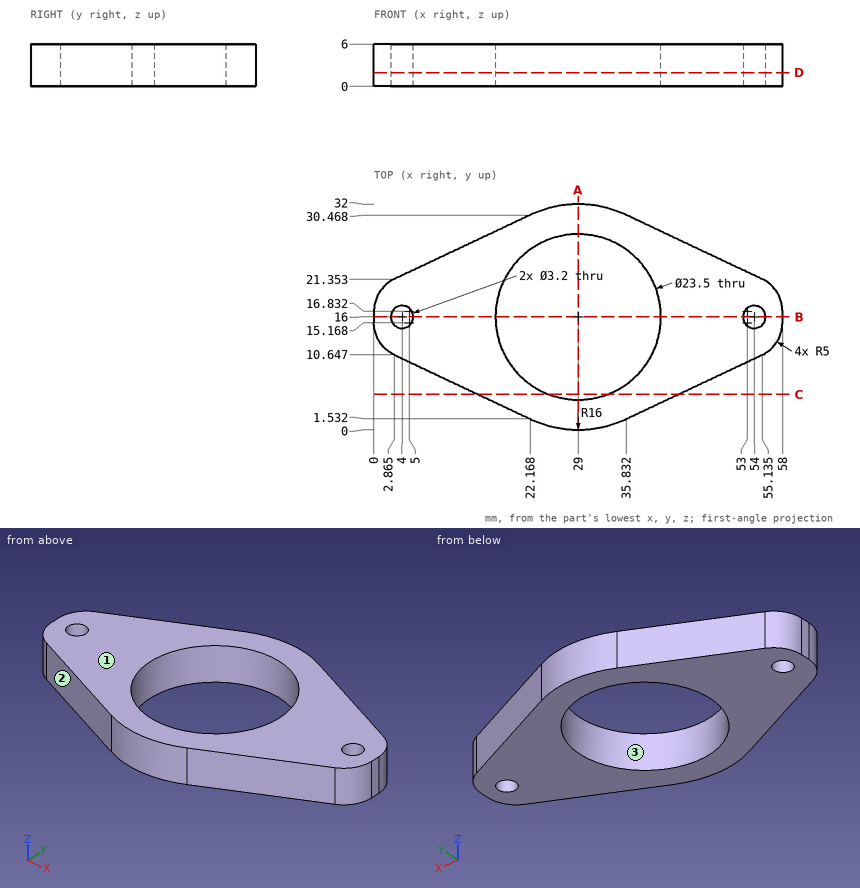
Geometry: see drawing. Coordinates: mm, zero at the bounding-box minimum. Give positions to 0.01 mm unless a question says otherwise; leave off trailing zeros. Order: outer loops, then holes, each group sorted by start corner. A loop starts at its lowest first (then second) coordinate and runs counter-clockwise, first axis right, second up. Notation, with made-up numbers: M 83,-15 L 96,-15 A23 ccw 96,11 Z; hole C 75,-9 d10. An arc over 180 degrees is marked long. Answer as a JSON object with one key per item and string values.
1. Cut plane D-D, the plane z = 1.95. State how many separate pieces and enclosed holes the cut face has.
Result sheet:
{"separate pieces": "1", "enclosed holes": "3"}
2. Pull-direction query (X, two-part tool) for the marked faces 1, 2 and 3; classes: +X half, -X half, draft (parallel to the pull), parting line (faces both ways), or undercut.
Result sheet:
{"face 1": "draft", "face 2": "-X half", "face 3": "undercut"}
3. Cut plane C-C, the plane y = 5. Output: boundary loops of the cut face in (x, z).
Result sheet:
{"outline": "M 14.82,0 L 24.87,0 L 24.87,6 L 14.82,6 Z; M 33.13,0 L 43.18,0 L 43.18,6 L 33.13,6 Z"}
4. Ray query, line 1 (Y direction, x = 54, z = 3.6); line 2 (Y direction, x = 33.5, z = 5.4) (1 decimal); line 3 (X direction, y = 8, z = 3.65) (1 decimal). Return the intervals inside material, ascending. Write a range as [from, to].
Result sheet:
{"line 1": "[10.11, 14.4], [17.6, 21.89]", "line 2": "[0.6, 5.1], [26.9, 31.4]", "line 3": "[8.5, 20.4], [37.6, 49.5]"}
5. Cut plane A-A, the plane x = 29. Output: boundary loops of the cut face in (y, z).
Result sheet:
{"outline": "M 0,0 L 4.25,0 L 4.25,6 L 0,6 Z; M 27.75,0 L 32,0 L 32,6 L 27.75,6 Z"}
6. First-contact query: P1, Ø2, axis at x = 38.5, z = 5.5, coming from the -Y side; P2, Ø2, axis at x = 51, z = 2.5, coming from the +Y side; P3, Ø1, axis at x = 38.5, z = 3, coming from the +Y side (1 decimal). Flat tips, straight axial feed; report the tip coordinate or a pass-through.
Result sheet:
{"P1": "y = 2.32", "P2": "y = 23.78", "P3": "y = 29.4"}
7. Cut plane B-B, the plane y = 16. Output: boundary loops of the cut face in (x, z), and give its area (3 significant figures).
Result sheet:
{"outline": "M 0,0 L 2.4,0 L 2.4,6 L 0,6 Z; M 5.6,0 L 17.25,0 L 17.25,6 L 5.6,6 Z; M 40.75,0 L 52.4,0 L 52.4,6 L 40.75,6 Z; M 55.6,0 L 58,0 L 58,6 L 55.6,6 Z", "area": "169 mm²"}
